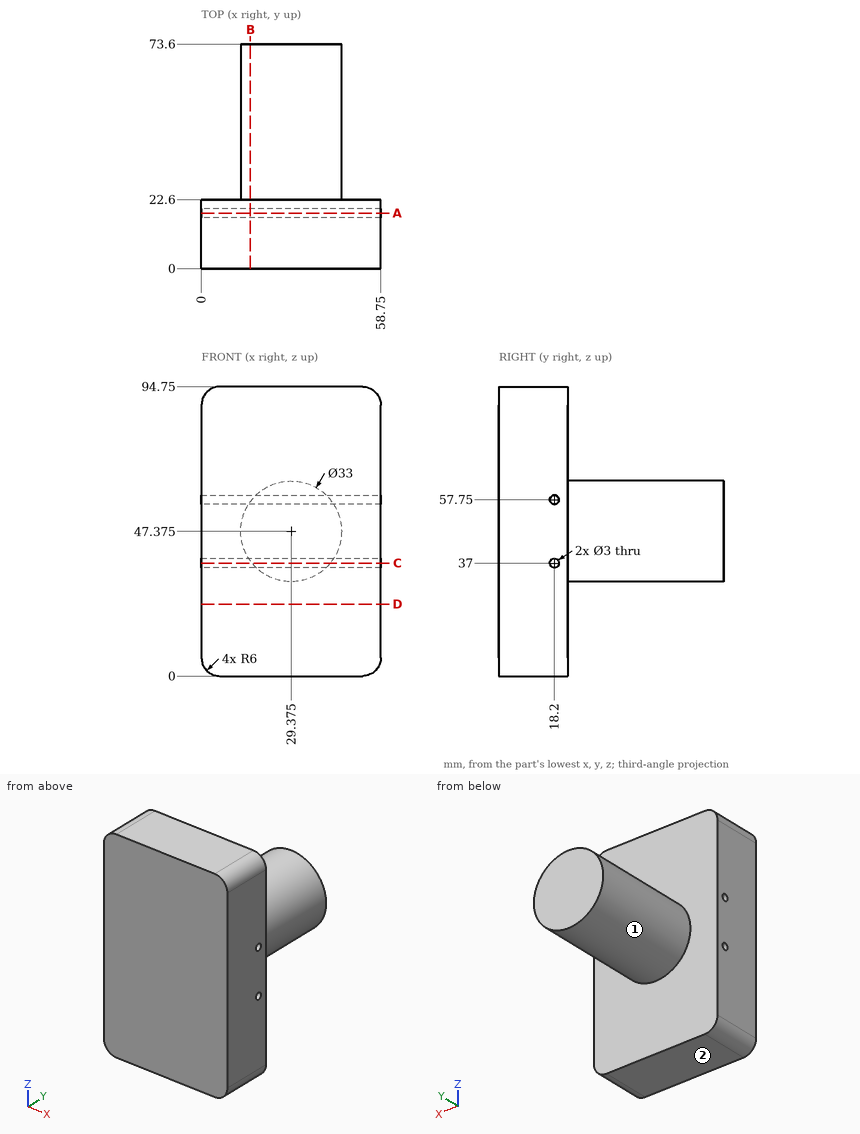
Geometry: see drawing. Coordinates: mm, zero at the bounding-box minimum. A direction names the side the tool comes from. Give positions to 0.01 mm unless a question says otherwise; leave off trailing zeros. Order: outer loops, then holes, each group sorted by start corner. A loop starts at its lowest first (then second) coordinate and runs counter-clockwise, first axis right, second up. Notation, with made-up numbers: M 74.5,46.5 L 115.5,46.5 A24 cw 115.5,72.5 Z; hole C 16.5,11 d4. An arc over 180 degrees is marked long. Answer as CSV lines item,"result". Start each with the question number.
1) Cut plane D-D (z = 23.5). Output: boundary loops of the cut face in (x, y).
2) First-contact query: P1, Ø1.5, axis at x = 44.5, y = 10, coming from the -Z side; P2, Ø8, axis at x = 24.5, y = 59, coming from the -Z side; P3, Ø12, axis at y = 62, z = 41, coming from the -X side. Flat tips, straight axial feed; report the tip coordinate or a pass-through.
3) Line query: line 1 (Y direction, x = 37, z = 37); line 2 (Z direction, x = 56, y = 19.5); line 3 (Y direction, x = 16, z = 37). Output: solid intervals per line, ascending. Write a range as from..to.
4) Cut plane A-A (y = 18.2). Output: boundary loops of the cut face in (x, z), then the cut area to 3 significant figures.
5) Cut plane C-C (z = 37). Output: boundary loops of the cut face in (x, y).
6) Set-up query: the marked faces 1 and 2. Return all of +Z, -Z, +X, -X, +Y, -Y with unobstructed straight access to the full face (end or side cutting, diameter ignored); none if empty.
7) Cut plane B-B (x = 16). Output: boundary loops of the cut face in (y, z).
Findings below:
1,outline,"M 0,0 L 58.75,0 L 58.75,22.6 L 0,22.6 Z"
2,P1,"stops at z = 0"
2,P2,"stops at z = 30.9"
2,P3,"stops at x = 12.88"
3,line 1,"y = 0..16.7, 19.7..73.6"
3,line 2,"z = 0.96..36.25, 37.75..57, 58.5..93.79"
3,line 3,"y = 0..16.7, 19.7..22.6"
4,outline,"M 0,6 A6 ccw 6,0 L 52.75,0 A6 ccw 58.75,6 L 58.75,35.5 L 0,35.5 Z; M 0,38.5 L 58.75,38.5 L 58.75,56.25 L 0,56.25 Z; M 0,59.25 L 58.75,59.25 L 58.75,88.75 A6 ccw 52.75,94.75 L 6,94.75 A6 ccw 0,88.75 Z"
4,area,"5,180 mm²"
5,outline,"M 0,0 L 58.75,0 L 58.75,16.7 L 0,16.7 Z; M 0,19.7 L 58.75,19.7 L 58.75,22.6 L 42.21,22.6 L 42.21,73.6 L 16.54,73.6 L 16.54,22.6 L 0,22.6 Z"
6,face 1,"+Y"
6,face 2,"-Z, +X, -X, +Y, -Y"
7,outline,"M 0,0 L 22.6,0 L 22.6,37.71 L 73.6,37.71 L 73.6,57.04 L 22.6,57.04 L 22.6,94.75 L 0,94.75 Z; hole C 18.2,37 d3; hole C 18.2,57.75 d3"
